```python
from build123d import *

# Parameters (mm, degrees)
BOSS_EXTRUDE1_DEPTH = 5
SKETCH3_R           = 1.5
CUT_EXTRUDE3_DEPTH  = 10


with BuildPart() as part:
    # Sketch1 → Boss-Extrude1 (new body)
    with BuildSketch(Plane(origin=(0, 0, 0), x_dir=(1, 0, 0), z_dir=(0, 1, 0))):
        Polygon((-77.5, 60), (-52.5, 60), (-52.5, 65), (-22.5, 65), (-22.5, 60), (22.5, 60), (22.5, 65), (52.5, 65), (52.5, 60), (77.5, 60), (77.5, 40), (82.5, 40), (82.5, 20), (77.5, 20), (77.5, -20), (82.5, -20), (82.5, -40), (77.5, -40), (77.5, -60), (52.5, -60), (52.5, -65), (22.5, -65), (22.5, -60), (-22.5, -60), (-22.5, -65), (-52.5, -65), (-52.5, -60), (-77.5, -60), (-77.5, -40), (-82.5, -40), (-82.5, -20), (-77.5, -20), (-77.5, 20), (-82.5, 20), (-82.5, 40), (-77.5, 40), align=None)
    extrude(amount=BOSS_EXTRUDE1_DEPTH)

    # Sketch3 → Cut-Extrude3 (cut)
    with BuildSketch(Plane(origin=(0, 5, 0), x_dir=(1, 0, 0), z_dir=(0, 1, 0))):
        with Locations(Location((-33.5, 32, 0), (0, 0, 270))):
            Circle(SKETCH3_R)
        with Locations(Location((32.5, -30, 0), (0, 0, 270))):
            Circle(SKETCH3_R)
        with BuildLine():
            Line((17.5, -25.666666667), (-17.5, -25.666666667))
            ThreePointArc((-17.5, -25.666666667), (-24.571067812, -22.737734479), (-27.5, -15.666666667))
            Line((-27.5, -15.666666667), (-27.5, 15.666666667))
            ThreePointArc((-27.5, 15.666666667), (-24.571067812, 22.737734479), (-17.5, 25.666666667))
            Line((-17.5, 25.666666667), (17.5, 25.666666667))
            ThreePointArc((17.5, 25.666666667), (24.571067812, 22.737734479), (27.5, 15.666666667))
            Line((27.5, 15.666666667), (27.5, -15.666666667))
            ThreePointArc((27.5, -15.666666667), (24.571067812, -22.737734479), (17.5, -25.666666667))
        make_face()
    extrude(amount=-CUT_EXTRUDE3_DEPTH, mode=Mode.SUBTRACT)


solid = part.part
```
Work out the finished part from the listing and answer in its coordinate system (mm). A direction names the side the tool comes from. Give positions to 0.01 mm unless a question says otherwise; leave off trailing zeros. Order: outer loops, then holes, each group sorted by start corner. A loop starts at its lowest first (then second) coordinate and runs counter-clockwise, first axis right, second up. Notation, with made-up numbers: (1, 69.5) - (29, 69.5) arc R28 cw to (29, 108.5) - close; hole circle Ø10 at (15, 84). An arc over 180 degrees is marked (long way). One line per item, written item: value. Start each with the question number.
1. Section D-D, the plane x = 62.5 is taken. Write down the section's boundary in (y, z), then the cut area to 3 significant figures.
2. Section A-A, the plane z = -13.5 is taken. Write down the section's boundary in (x, y).
3. Consider line 1 (X direction, y = 1.35, z = 16); line 2 (X direction, y = 2.3, z = -32); line 3 (Z direction, x = 14, y = 3.75). Determine where each line is inside the solid, lowest interval first.
4. Section C-C, the plane y = 1.05 is taken. Count the separate pieces of the cut face and the enclosed holes in it, then the cut area to 3 significant figures.
5. Which of the six approach directions +Z, -Z, +X, -X, +Y, -Y give full straight-line access (tool end or side, diameter ignored) to faces 1 (the face through (-77.5, 2, 50)), 2 (the face through (65, 2, -60)), 3 (the face through (22.5, 2, 63))?
6. For a pull along Z with two mould halves and no side action, classify faces 4 (the face through (27.5, 3, 0)), 5 (the face through (52.5, 2, 62)), 6 (the face through (37, 2, -65)) as released by +Z, released by -Z, zero draft, split by the parting line, or undercut.
7. Section B-B, the plane x = -2 is taken. Write down the section's boundary in (y, z), then the cut area to 3 significant figures.
8. Each of these flat-tipped pins is pushed along its axis until it touches: pin 1 Ø4 at (x, z) = (-33.5, -32) entering from -Y; pin 2 Ø2.5 at (y, z) = (1.5, 3.5) entering from +X; pin 3 Ø2.5 at (x, y) = (-2, 3.5) entering from -Z; pin 4 Ø12 at (x, z) = (19.5, 12) entering from -Y. Where does it stop, or does it pass through?
Filled sheet:
1. outline: (0, -60) - (5, -60) - (5, 60) - (0, 60) - close
1. area: 600 mm²
2. outline: (-77.5, 0) - (-27.5, 0) - (-27.5, 5) - (-77.5, 5) - close; (27.5, 0) - (77.5, 0) - (77.5, 5) - (27.5, 5) - close
3. line 1: -77.5 to -27.49, 27.49 to 77.5
3. line 2: -82.5 to -35, -32 to 82.5
3. line 3: -60 to -25.67, 25.67 to 60
4. separate pieces: 1
4. enclosed holes: 3
4. area: 16,800 mm²
5. face 1: +Z, -X, +Y, -Y
5. face 2: -Z, +X, +Y, -Y
5. face 3: +Z, +Y, -Y
6. face 4: undercut
6. face 5: zero draft
6. face 6: released by -Z
7. outline: (0, -60) - (5, -60) - (5, -25.67) - (0, -25.67) - close; (0, 25.67) - (5, 25.67) - (5, 60) - (0, 60) - close
7. area: 343 mm²
8. pin 1: y = 0
8. pin 2: x = 77.5
8. pin 3: z = -60
8. pin 4: through
